```python
from build123d import *

# Parameters (mm, degrees)
S01_CENTRAL_SPINDLE_PAD_R         = 13
F_01_CENTRAL_SPINDLE_PAD_DEPTH    = 8
F_02_CAGE_RIB_1_DEPTH             = 8
F_03_CAGE_RIB_2_DEPTH             = 8
F_04_CAGE_RIB_3_DEPTH             = 8
F_05_START                        = -1
S05_THREE_CAGE_BOLT_HOLES_R       = 3.3
F_05_THREE_CAGE_BOLT_HOLES_DEPTH  = 10
F_06_START                        = -1
S06_SPINDLE_STEM_CLEARANCE_R      = 5.3
F_06_SPINDLE_STEM_CLEARANCE_DEPTH = 10


with BuildPart() as part:
    # S01 - Central spindle pad → 01 - Central spindle pad (new body)
    with BuildSketch(Plane.XY):
        Circle(S01_CENTRAL_SPINDLE_PAD_R)
    extrude(amount=F_01_CENTRAL_SPINDLE_PAD_DEPTH)

    # S02 - Cage rib 1 → 02 - Cage rib 1 (add)
    with BuildSketch(Plane.XY):
        with BuildLine():
            Line((-8.5, 0), (-8.5, 54))
            ThreePointArc((-8.5, 54), (0, 62.5), (8.5, 54))
            Line((8.5, 54), (8.5, 0))
            ThreePointArc((8.5, 0), (0, -8.5), (-8.5, 0))
        make_face()
    extrude(amount=F_02_CAGE_RIB_1_DEPTH)

    # S03 - Cage rib 2 → 03 - Cage rib 2 (add)
    with BuildSketch(Plane.XY):
        with BuildLine():
            Line((0, -8.5), (-54, -8.5))
            ThreePointArc((-54, -8.5), (-62.5, 0), (-54, 8.5))
            Line((-54, 8.5), (0, 8.5))
            ThreePointArc((0, 8.5), (8.5, 0), (0, -8.5))
        make_face()
    extrude(amount=F_03_CAGE_RIB_2_DEPTH)

    # S04 - Cage rib 3 → 04 - Cage rib 3 (add)
    with BuildSketch(Plane.XY):
        with BuildLine():
            Line((8.5, 0), (8.5, -54))
            ThreePointArc((8.5, -54), (0, -62.5), (-8.5, -54))
            Line((-8.5, -54), (-8.5, 0))
            ThreePointArc((-8.5, 0), (0, 8.5), (8.5, 0))
        make_face()
    extrude(amount=F_04_CAGE_RIB_3_DEPTH)

    # S05 - Three cage bolt holes → 05 - Three cage bolt holes (cut)
    with BuildSketch(Plane.XY.offset(F_05_START)):
        with Locations((0, 54)):
            Circle(S05_THREE_CAGE_BOLT_HOLES_R)
        with Locations((-54, 0)):
            Circle(S05_THREE_CAGE_BOLT_HOLES_R)
        with Locations((0, -54)):
            Circle(S05_THREE_CAGE_BOLT_HOLES_R)
    extrude(amount=F_05_THREE_CAGE_BOLT_HOLES_DEPTH, mode=Mode.SUBTRACT)

    # S06 - Spindle stem clearance → 06 - Spindle stem clearance (cut)
    with BuildSketch(Plane.XY.offset(F_06_START)):
        Circle(S06_SPINDLE_STEM_CLEARANCE_R)
    extrude(amount=F_06_SPINDLE_STEM_CLEARANCE_DEPTH, mode=Mode.SUBTRACT)


solid = part.part
```
CAD build for the part. Positions are in the model's coordinates, mm. A direction names the side the tool comes from. Give positions to 0.01 mm unless a question says otherwise; leave off trailing zeros. Loops run counter-clockwise (first coordinate to the right, second up) from the corner with the lowest first, then second, coordinate; pieces in that order, holes last. Notation, with made-up numbers: M -31,59.5 L 24,59.5 A16 cw 24,89.5 Z; hole C 58,53.5 d7. An arc over 180 degrees is marked long. Use one line per item in the form item = value.
Item 1: Two-plate mould, pull along Y, no slides. Class faces 6 (the face through (-62.498, -0.187, 3.944)), 7 (the face through (8.5, -32, 4)), 8 (the face through (4.896, -2.03, 3.944)): pulls with the +Y half, pulls with the -Y half, needs draft (parallel to the pull), parting line crosses it, or undercut.
Determined:
face_6 = parting line crosses it
face_7 = needs draft
face_8 = undercut
Item 2: Slice it at C-C (y = 0). List the corners of the cut face in (x, z).
Determined:
outline = M -62.5,0 L -57.3,0 L -57.3,8 L -62.5,8 Z; M -50.7,0 L -5.3,0 L -5.3,8 L -50.7,8 Z; M 5.3,0 L 13,0 L 13,8 L 5.3,8 Z
Item 3: Slice it at D-D (x = -25). List the corners of the cut face in (y, z), plus the area to 3 significant figures.
Determined:
outline = M -8.5,0 L 8.5,0 L 8.5,8 L -8.5,8 Z
area = 136 mm2
Item 4: Flat gauge pins, fed straight in: pin 1 (2.5 mm diameter, centred on x = -34, z = 4.5, fed in from -Y); pin 2 (8.5 mm diameter, centred on x = 0, y = 54, fed in from +Z); pin 3 (4 mm diameter, centred on y = 4, z = 2.5, fed in from -X); pin 4 (1.5 mm diameter, centred on y = 4.5, z = 4.5, fed in from -X). Where does each tip first touch, or does it go through?
Determined:
pin_1 = -8.5
pin_2 = 8
pin_3 = -62.26
pin_4 = -61.63
Item 5: Slice it at A-A (x = 0). List the corners of the cut face in (y, z), plus the area to 3 significant figures.
Determined:
outline = M -62.5,0 L -57.3,0 L -57.3,8 L -62.5,8 Z; M -50.7,0 L -5.3,0 L -5.3,8 L -50.7,8 Z; M 5.3,0 L 50.7,0 L 50.7,8 L 5.3,8 Z; M 57.3,0 L 62.5,0 L 62.5,8 L 57.3,8 Z
area = 810 mm2
Item 6: Slice it at B-B (z = 6). List the corners of the cut face in (x, y), plus the area to 3 significant figures.
Determined:
outline = M -54,-8.5 L -9.84,-8.5 A13 ccw -8.5,-9.84 L -8.5,-54 A8.5 ccw 8.5,-54 L 8.5,-9.84 A13 ccw 8.5,9.84 L 8.5,54 A8.5 ccw -8.5,54 L -8.5,9.84 A13 ccw -9.84,8.5 L -54,8.5 A8.5 ccw Z; hole C -54,0 d6.6; hole C 0,0 d10.6; hole C 0,-54 d6.6; hole C 0,54 d6.6
area = 2,820 mm2
Item 7: Drill centre lines: probe 1 along Y at (x, z) = (0, 5.25); probe 2 along X at (y, z) = (0, 3.5); probe 3 along X at (y, z) = (54, 4.25). Where is each one in solid material? Low to high. Write a range as from..to.
Determined:
probe_1 = -62.5..-57.3, -50.7..-5.3, 5.3..50.7, 57.3..62.5
probe_2 = -62.5..-57.3, -50.7..-5.3, 5.3..13
probe_3 = -8.5..-3.3, 3.3..8.5
Item 8: Which spindle directions (+Z, -Z, +X, -X, +Y, -Y) get a long thin tool onto all of the face, cutting with end or side? Do faces 1 (the face through (0.187, -62.498, 3.944)), 2 (the face through (13, 0, 4)), 3 (the face through (-8.5, -32, 4)), 4 (the face through (8.5, 32, 4)), 5 (the face through (-8.5, 32, 4)). Say none if no direction does.
Determined:
face_1 = +Z, -Z, -Y
face_2 = +Z, -Z, +X
face_3 = +Z, -Z, -X, -Y
face_4 = +Z, -Z, +X, +Y
face_5 = +Z, -Z, -X, +Y
